from build123d import *

# Parameters (mm, degrees)
BOSS_EXTRUDE1_DEPTH = 3
SKETCH2_R           = 1
CUT_EXTRUDE1_DEPTH  = 10


with BuildPart() as part:
    # Sketch1 → Boss-Extrude1 (new body)
    with BuildSketch(Plane(origin=(0, 0, 0), x_dir=(1, 0, 0), z_dir=(0, 1, 0))):
        Polygon((4.9, 17), (4.9, 21.75), (14.9, 21.75), (14.9, 17), (23.75, 17), (23.75, -17), (14.9, -17), (14.9, -21.75), (4.9, -21.75), (4.9, -17), (-4.9, -17), (-4.9, -21.75), (-14.9, -21.75), (-14.9, -17), (-23.75, -17), (-23.75, 17), (-14.9, 17), (-14.9, 21.75), (-4.9, 21.75), (-4.9, 17), align=None)
    extrude(amount=BOSS_EXTRUDE1_DEPTH)

    # Sketch2 → Cut-Extrude1 (cut)
    with BuildSketch(Plane(origin=(0, 3, 0), x_dir=(1, 0, 0), z_dir=(0, 1, 0))):
        with Locations(Location((-21.25, 8.75, 0), (0, 0, 270))):
            Circle(SKETCH2_R)
        with Locations(Location((-21.25, -8.75, 0), (0, 0, 270))):
            Circle(SKETCH2_R)
        with Locations(Location((21.25, -8.75, 0), (0, 0, 270))):
            Circle(SKETCH2_R)
        with Locations(Location((21.25, 8.75, 0), (0, 0, 270))):
            Circle(SKETCH2_R)
    extrude(amount=-CUT_EXTRUDE1_DEPTH, mode=Mode.SUBTRACT)


solid = part.part
Here's how the part is built. I have some questions about the finished solid (model axes, mm). A direction names the side the tool comes from. Coordinates: 2 decimals unless noted, no trailing zeros. Write each loop counter-clockwise with the first axis right and the second up, starting at its lowest first coordinate (ties: lowest second). Pieces come first, ordered by that corner, then holes. Notation, with made-up numbers: (12.5, -32.5) - (66.5, -32.5) arc R34 cw to (66.5, -1.5) - close; hole circle Ø10 at (-29, 19). An arc over 180 degrees is marked (long way). Use one line per item in the form item = value.
1) Suppose I cut it at D-D, the plane z = -8.75. Write out the boundary of the cut face in (x, y), plus the area to 4 significant figures.
Solved:
outline = (-23.75, 0) - (-22.25, 0) - (-22.25, 3) - (-23.75, 3) - close; (-20.25, 0) - (20.25, 0) - (20.25, 3) - (-20.25, 3) - close; (22.25, 0) - (23.75, 0) - (23.75, 3) - (22.25, 3) - close
area = 130.5 mm2
2) Suppose I cut it at A-A, the plane x = -21.25. Write out the boundary of the cut face in (y, z).
Solved:
outline = (0, -17) - (3, -17) - (3, -9.75) - (0, -9.75) - close; (0, -7.75) - (3, -7.75) - (3, 7.75) - (0, 7.75) - close; (0, 9.75) - (3, 9.75) - (3, 17) - (0, 17) - close
3) I'm going to push flat-ended pins straight in: P1, Ø0.9, axis at x = 21.5, y = 2, coming from the +Z side; P2, Ø1.5, axis at x = 17.5, y = 2, coming from the -Z side; P3, Ø1.2, axis at x = 21.25, z = 8.75, coming from the +Y side; P4, Ø2.5, axis at x = 21.25, z = -8.75, coming from the -Y side. Where does each tip first touch, or does it pass through?
Solved:
P1 = 17
P2 = -17
P3 = through
P4 = 0
4) I need wall thicknesses on line 1 (X direction, y = 1.55, z = 8.75); line 2 (X direction, y = 0.6, z = 18); line 3 (Z direction, x = 2, y = 2.15). Which ranges of each line are inside material? Lowest first, please.
Solved:
line_1 = -23.75 to -22.25, -20.25 to 20.25, 22.25 to 23.75
line_2 = -14.9 to -4.9, 4.9 to 14.9
line_3 = -17 to 17
5) Suppose I cut it at C-C, the plane y = 0.6. Write out the boundary of the cut face in (x, z).
Solved:
outline = (-23.75, -17) - (-14.9, -17) - (-14.9, -21.75) - (-4.9, -21.75) - (-4.9, -17) - (4.9, -17) - (4.9, -21.75) - (14.9, -21.75) - (14.9, -17) - (23.75, -17) - (23.75, 17) - (14.9, 17) - (14.9, 21.75) - (4.9, 21.75) - (4.9, 17) - (-4.9, 17) - (-4.9, 21.75) - (-14.9, 21.75) - (-14.9, 17) - (-23.75, 17) - close; hole circle Ø2 at (-21.25, -8.75); hole circle Ø2 at (-21.25, 8.75); hole circle Ø2 at (21.25, -8.75); hole circle Ø2 at (21.25, 8.75)
6) Suppose I cut it at B-B, the plane z = -18.5. Write out the boundary of the cut face in (x, y).
Solved:
outline = (-14.9, 0) - (-4.9, 0) - (-4.9, 3) - (-14.9, 3) - close; (4.9, 0) - (14.9, 0) - (14.9, 3) - (4.9, 3) - close
7) On a 3-axis mill with a long thin cutter (end or side, diameter ignored), from which of +Z, -Z, +X, -X, +Y, -Y can I reach the whole of each face in a straight line? I mean faces 4 (the flat face through (4.9, 1, 19)), 5 (the flat face through (10, 1, -21.75)), 6 (the flat face through (-19, 1, -17)), 7 (the flat face through (19, 1, -17)), 8 (the flat face through (-19, 1, 17)). Say none if no direction works.
Solved:
face_4 = +Z, +Y, -Y
face_5 = -Z, +X, -X, +Y, -Y
face_6 = -Z, -X, +Y, -Y
face_7 = -Z, +X, +Y, -Y
face_8 = +Z, -X, +Y, -Y
8) Thinking about a two-plate mould opening in X: for faces 1 (the flat face through (4.9, 1, -19)), 2 (the flat face through (19, 1, 17)), 3 (the flat face through (0, 1, -17)), which applies, released by +X, released by -X, zero draft, split by the parting line, or undercut?
Solved:
face_1 = undercut
face_2 = zero draft
face_3 = undercut
